Design review of the part built by this model. Coordinates are the model's own, in mm. A direction names the side the tool comes from. Give positions to 0.01 mm unless a question says otherwise; leave off trailing zeros. Loops run counter-clockwise (first coordinate to the right, second up) from the corner with the lowest first, then second, coordinate; pieces in that order, holes last.
from build123d import *

# Parameters (mm, degrees)
SALIENTE_EXTRUIR1_DEPTH = 1.6
CROQUIS2_R              = 3.45
SALIENTE_EXTRUIR2_DEPTH = 1.4
CORTAR_EXTRUIR1_REACH   = 20.276
CROQUIS3_R              = 2.1


with BuildPart() as part:
    # Croquis1 → Saliente-Extruir1 (new body)
    with BuildSketch(Plane(origin=(0, 0, 0), x_dir=(1, 0, 0), z_dir=(0, 1, 0))):
        with BuildLine():
            Line((1, 0), (14, 0))
            ThreePointArc((14, 0), (14.707106781, 0.292893219), (15, 1))
            Line((15, 1), (15, 9))
            ThreePointArc((15, 9), (14.707106781, 9.707106781), (14, 10))
            Line((14, 10), (1, 10))
            ThreePointArc((1, 10), (0.292893219, 9.707106781), (0, 9))
            Line((0, 9), (0, 1))
            ThreePointArc((0, 1), (0.292893219, 0.292893219), (1, 0))
        make_face()
    extrude(amount=SALIENTE_EXTRUIR1_DEPTH)

    # Croquis2 → Saliente-Extruir2 (add)
    with BuildSketch(Plane(origin=(0, 1.6, 0), x_dir=(1, 0, 0), z_dir=(0, 1, 0))):
        with Locations(Location((7.5, 5, 0), (0, 0, 90))):
            Circle(CROQUIS2_R)
    extrude(amount=SALIENTE_EXTRUIR2_DEPTH)

    # Croquis3 → Cortar-Extruir1 (cut, up to next)
    with BuildSketch(Plane(origin=(0, 3, 0), x_dir=(1, 0, 0), z_dir=(0, 1, 0)), mode=Mode.PRIVATE) as cortar_extruir1_sk1:
        with Locations(Location((7.5, 5, 0), (0, 0, 270))):
            Circle(CROQUIS3_R)
    cortar_extruir1_tool1 = extrude(cortar_extruir1_sk1.sketch, amount=-CORTAR_EXTRUIR1_REACH, mode=Mode.PRIVATE) & part.part
    add(cortar_extruir1_tool1.solids().sort_by_distance((7.5, 3, -5))[0], mode=Mode.SUBTRACT)


solid = part.part
Q1. Take a section at D-D (x = 11.5). Give the boundary of the cut face in (y, z), plus the area to 3 significant figures.
Results:
outline: (0, -10) - (1.6, -10) - (1.6, 0) - (0, 0) - close
area: 16.0 mm2
Q2. Tool access review of faces 4 (the face through (15, 1, -5)), 5 (the face through (4, 1.6, -6)): name each direction out of +Z, -Z, +X, -X, +Y, -Y from which nothing blocks a thin tool from reaching the whole face with its end or side.
Results:
face 4: +Z, -Z, +X, +Y, -Y
face 5: +Y
Q3. Take a section at C-C (y = 0.4). Give the boundary of the cut face in (x, z), plus the area to 3 significant figures.
Results:
outline: (0, -9) arc R1 ccw to (1, -10) - (14, -10) arc R1 ccw to (15, -9) - (15, -1) arc R1 ccw to (14, 0) - (1, 0) arc R1 ccw to (0, -1) - close; hole circle Ø4.2 at (7.5, -5)
area: 135 mm2
Q4. Draft analysis for pull direction X (two halves, no side actions). For faces 1 (the face through (9.599, 2.29, -2.262)), 2 (the face through (9.582, 1.521, -5.273)), 3 (the face through (0.285, 0.789, -0.301)), state which applies: pulls with the +X half, pulls with the -X half, needs draft (parallel to the pull), parting line crosses it, or undercut.
Results:
face 1: parting line crosses it
face 2: undercut
face 3: pulls with the -X half
Q5. Take a section at A-A (z = -5). Give the boundary of the cut face in (x, y), plus the area to 3 significant figures.
Results:
outline: (0, 0) - (5.4, 0) - (5.4, 3) - (4.05, 3) - (4.05, 1.6) - (0, 1.6) - close; (9.6, 0) - (15, 0) - (15, 1.6) - (10.95, 1.6) - (10.95, 3) - (9.6, 3) - close
area: 21.1 mm2
Q6. Take a section at B-B (x = 7.5). Give the boundary of the cut face in (y, z), plus the area to 3 significant figures.
Results:
outline: (0, -10) - (1.6, -10) - (1.6, -8.45) - (3, -8.45) - (3, -7.1) - (0, -7.1) - close; (0, -2.9) - (3, -2.9) - (3, -1.55) - (1.6, -1.55) - (1.6, 0) - (0, 0) - close
area: 13.1 mm2
Q7. Wall thickness on line 1 (X direction, y = 1.2, z = -5); line 2 (X direction, y = 2.3, z = -5); line 3 (Y direction, x = 1.75, z = -7): over which ranges is each line inside the solid? List them lowest first.
Results:
line 1: x = 0 to 5.4, 9.6 to 15
line 2: x = 4.05 to 5.4, 9.6 to 10.95
line 3: y = 0 to 1.6
